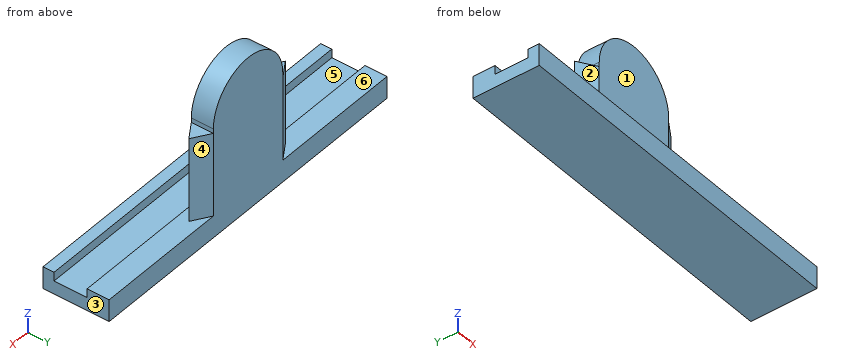
```python
from build123d import *

# Parameters (mm, degrees)
F1_DEPTH = 6.35
F3_DEPTH = 24.13
F4_W     = 101.6
F4_H     = 6.35
F5_DEPTH = 6.35
F7_DEPTH = 12.7
F8_W     = 9.525
F8_H     = 2.54
F9_DEPTH = 114.282591


with BuildPart() as f1:
    # F0 (on Front) → F1 (new body)
    with BuildSketch(Plane.XZ):
        with BuildLine():
            Line((0, 25.4), (0, 0))
            Line((0, 0), (25.4, 0))
            Line((25.4, 0), (25.4, 25.4))
            ThreePointArc((25.4, 25.4), (12.7, 38.1), (0, 25.4))
        make_face()
    extrude(amount=F1_DEPTH)

    # F2 (on face) → F3 (join)
    with BuildSketch(Plane(origin=(0, 0, 0), x_dir=(1, 0, 0), z_dir=(0, 0, -1))):
        Polygon((-4.953, 3.175), (0, 0), (0, 6.35), align=None)
        Polygon((30.353, 3.175), (25.4, 6.35), (25.4, 0), align=None)
    extrude(amount=-F3_DEPTH)

    # F4 (on face) → F5 (join)
    with BuildSketch(Plane(origin=(0, 0, 0), x_dir=(1, 0, 0), z_dir=(0, 0, -1))):
        with Locations((12.7, 3.175)):
            Rectangle(F4_W, F4_H)
    extrude(amount=F5_DEPTH)

    # F6 (on face) → F7 (join)
    with BuildSketch(Plane.XZ.offset(6.35)):
        Polygon((25.4, 0), (0, 0), (-38.1, 0), (-38.1, -6.35), (63.5, -6.35), (63.5, 0), align=None)
    extrude(amount=F7_DEPTH)

    # F8 (on face) → F9 (cut)
    with BuildSketch(Plane.YZ.offset(63.5)):
        with Locations((-11.1125, -1.27)):
            Rectangle(F8_W, F8_H)
    extrude(amount=-F9_DEPTH, mode=Mode.SUBTRACT)


solid = f1.part
```
Check sheet for the modelled part. Datum: model origin and axes. Units: mm. Face numbers are marked on the shaded views. A direction names the side the tool comes from. Coordinates: 2 decimals unless noted, no trailing zeros. Write each loop counter-clockwise with the first axis right and the second up, starting at its lowest first coordinate (ties: lowest second). Pieces come first, ordered by that corner, then holes. Notation, with made-up numbers: (-20, -13) -> (0, -13) arc R23 cw to (0, 25) -> close; hole circle Ø4 at (77.25, -32). An arc over 180 degrees is marked (long way). Use a Markdown table: item, result.
1. Tool access check on the marked faces 1, 2 and 3. Record the directions out of +Z, -Z, +X, -X, +Y, -Y that give a thin tool (end or side, any length) a straight path to the whole face; none if there is none.
Reported:
| item | result |
|---|---|
| face 1 | +Z, +X, -X |
| face 2 | +Z, -X, -Y |
| face 3 | +Z, -Z, +X, +Y, -Y |
2. Release check for a two-part mould opening along Y. For the marked faces 4, 5 and 6 record: pulls with the +Y half, pulls with the -Y half, needs draft (parallel to the pull), parting line crosses it, or undercut.
Reported:
| item | result |
|---|---|
| face 4 | pulls with the +Y half |
| face 5 | undercut |
| face 6 | needs draft |
3. Scan lines: line 1 along Y through (x, z) = (39, -1) (3 decimals); line 2 along Y through (x, z) = (2, 20.5); line 3 along Z through (x, y) = (-10, -15). Record each from-to range of solid material in increasing order.
Reported:
| item | result |
|---|---|
| line 1 | y = -19.05 to -15.875, -6.35 to 0 |
| line 2 | y = -6.35 to 0 |
| line 3 | z = -6.35 to -2.54 |
4. Sectioned sample at D-D (x = 12.7). Enter the section's corners in (y, z) (3 decimals), plus the area to 3 significant figures.
Reported:
| item | result |
|---|---|
| outline | (-19.05, -6.35) -> (0, -6.35) -> (0, 38.1) -> (-6.35, 38.1) -> (-6.35, -2.54) -> (-15.875, -2.54) -> (-15.875, 0) -> (-19.05, 0) -> close |
| area | 339 mm2 |
5. Sectioned sample at B-B (z = 10). Enter the section's corners in (x, y) (3 decimals).
Reported:
| item | result |
|---|---|
| outline | (-4.953, -3.175) -> (0, -6.35) -> (25.4, -6.35) -> (30.353, -3.175) -> (25.4, 0) -> (0, 0) -> close |
6. Sectioned sample at C-C (y = -9.75). Enter the section's corners in (x, z).
Reported:
| item | result |
|---|---|
| outline | (-38.1, -6.35) -> (63.5, -6.35) -> (63.5, -2.54) -> (-38.1, -2.54) -> close |
7. Sectioned sample at A-A (x = -6.5). Enter the section's corners in (y, z) (3 decimals), plus the area to 3 significant figures.
Reported:
| item | result |
|---|---|
| outline | (-19.05, -6.35) -> (0, -6.35) -> (0, 0) -> (-6.35, 0) -> (-6.35, -2.54) -> (-15.875, -2.54) -> (-15.875, 0) -> (-19.05, 0) -> close |
| area | 96.8 mm2 |
8. Go/stop test with flat-tipped pins: pin 1 Ø1 at (x, z) = (-1.5, 6.5) entering from -Y; pin 2 Ø8 at (x, y) = (45, -5) entering from +Z; pin 3 Ø5 at (y, z) = (-4, 4.5) entering from -X. Record where each tip stops, or that it passes through.
Reported:
| item | result |
|---|---|
| pin 1 | stops at y = -5.71 |
| pin 2 | stops at z = 0 |
| pin 3 | stops at x = -4.95 |
